Work out the finished part from the listing and answer in its coordinate system (mm). Face numbers are marked on the shaded views. A direction names the side the tool comes from. Give positions to 0.01 mm unless a question says otherwise; leave off trailing zeros. Write each loop counter-clockwise with the first axis right and the second up, starting at its lowest first coordinate (ties: lowest second). Pieces come first, ordered by that corner, then holes.
1) Find section A-A (z = 4.85). Determine the outline of the cut face in (x, y), plus the area to 3 significant figures.
2) Straight lines are drawn through the part: probe 1 along Y at (x, z) = (13.25, 3); probe 2 along Y at (x, z) = (3, 4.65); probe 3 along X at (y, z) = (4, 4.9). For each, find the intervals that lie inside material, in ascending order.
3) Find section C-C (y = 4). Determine the outline of the cut face in (x, z), plus the area to 3 significant figures.
4) Given pin 1 Ø3.5 at (x, y) = (2.5, 3.5) entering from -Z; pin 2 Ø1.5 at (y, z) = (4, 3) entering from +X, each flat-ended and moving along its own axis, determine where each tip first touches the part or whether it passes through.
5) A tool of negligible diameter and unlimited length cuts with its end or side. For the marked faces 1 and 2, from which of +Z, -Z, +X, -X, +Y, -Y can it reach the whole face along a straight path? Write none if from no direction.
6) Find section B-B (x = 3). Determine the outline of the cut face in (y, z).
7) Determine the mould class of the marked faces 3, 4 and 5 for opening direction Y: pulls with the +Y half, pulls with the -Y half, needs draft (parallel to the pull), parting line crosses it, or undercut.
8) Find section D-D (x = 18.5). Determine the outline of the cut face in (y, z), plus the area to 3 significant figures.
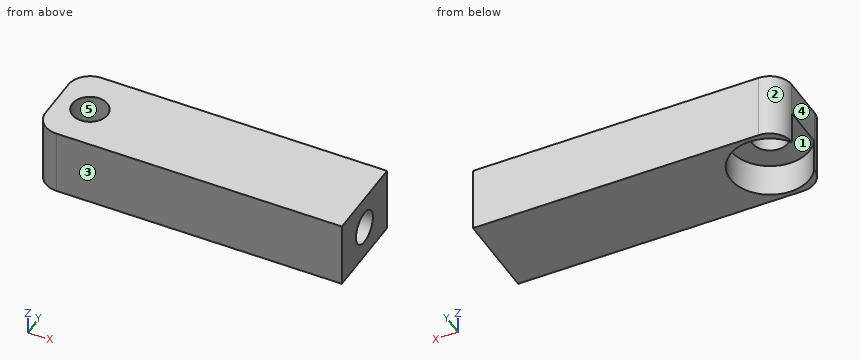
```python
from build123d import *

# Parameters (mm, degrees)
SKETCH_2_R          = 1.6
EXTRUDE_1_DEPTH     = 6
SKETCH_3_R          = 1.5
CUT_EXTRUDE_1_DEPTH = 20
SKETCH_4_R          = 3.6
CUT_EXTRUDE_2_DEPTH = 3


with BuildPart() as part:
    # 草图2 → 凸台-拉伸1 (new body)
    with BuildSketch(Plane.XY):
        with BuildLine():
            Line((0, 2), (0, 6))
            ThreePointArc((0, 6), (0.585786438, 7.414213562), (2, 8))
            Line((2, 8), (28, 8))
            Line((28, 8), (28, 0))
            Line((28, 0), (2, 0))
            ThreePointArc((2, 0), (0.585786438, 0.585786438), (0, 2))
        make_face()
        with Locations((3, 4)):
            Circle(SKETCH_2_R, mode=Mode.SUBTRACT)
    extrude(amount=EXTRUDE_1_DEPTH)

    # 草图3 → 切除-拉伸1 (cut)
    with BuildSketch(Plane(origin=(28, 0, 0), x_dir=(0, 0, -1), z_dir=(1, 0, 0))):
        with Locations((-3, 4)):
            Circle(SKETCH_3_R)
    extrude(amount=-CUT_EXTRUDE_1_DEPTH, mode=Mode.SUBTRACT)

    # 草图4 → 切除-拉伸2 (cut)
    with BuildSketch(Plane(origin=(0, 0, 0), x_dir=(-1, 0, 0), z_dir=(0, 0, -1))):
        with Locations((-3, 4)):
            Circle(SKETCH_4_R)
    extrude(amount=-CUT_EXTRUDE_2_DEPTH, mode=Mode.SUBTRACT)


solid = part.part
```
Results:
1. outline: (0, 2) arc R2 ccw to (2, 0) - (28, 0) - (28, 8) - (2, 8) arc R2 ccw to (0, 6) - close; hole circle Ø3.2 at (3, 4)
1. area: 214 mm2
2. probe 1: y = 0 to 2.5, 5.5 to 8
2. probe 2: y = 0 to 2.4, 5.6 to 8
2. probe 3: x = 0 to 1.4, 4.6 to 28
3. outline: (0, 3) - (1.4, 3) - (1.4, 6) - (0, 6) - close; (4.6, 3) - (6.6, 3) - (6.6, 0) - (28, 0) - (28, 1.5) - (8, 1.5) - (8, 4.5) - (28, 4.5) - (28, 6) - (4.6, 6) - close
3. area: 78.6 mm2
4. pin 1: stops at z = 3
4. pin 2: stops at x = 8
5. face 1: -Z
5. face 2: +Z, -Z, -X, +Y
6. outline: (0, 0) - (0.4, 0) - (0.4, 3) - (2.4, 3) - (2.4, 6) - (0, 6) - close; (5.6, 3) - (7.6, 3) - (7.6, 0) - (8, 0) - (8, 6) - (5.6, 6) - close
7. face 3: pulls with the -Y half
7. face 4: needs draft
7. face 5: undercut
8. outline: (0, 0) - (8, 0) - (8, 6) - (0, 6) - close; hole circle Ø3 at (4, 3)
8. area: 40.9 mm2
